```python
from build123d import *

# Parameters (mm, degrees)
TOP_DEPTH             = 5.08
SKETCH2_W             = 5.08
SKETCH2_H             = 44.45
BOLT_ATTACH_DEPTH     = 19.05
BOLTHOLES_LOWER_DEPTH = 5.08
MIRROREDFILLET_R      = 2.54
CENTERFILLET_R        = 6.35
CHAMFER1_SIZE         = 2.54


with BuildPart() as part:
    # Sketch1 → top (new body)
    with BuildSketch(Plane(origin=(0, 0, 0), x_dir=(1, 0, 0), z_dir=(0, 1, 0))):
        Polygon((0, 0), (0, 63.5), (7.62, 63.5), (7.62, 25.4), (17.78, 19.05), (17.78, 0), align=None)
        with BuildLine():
            Line((12.7, 13.97), (12.7, 7.62))
            ThreePointArc((12.7, 7.62), (8.89, 3.81), (5.08, 7.62))
            Line((5.08, 7.62), (5.08, 13.97))
            ThreePointArc((5.08, 13.97), (8.89, 17.78), (12.7, 13.97))
        make_face(mode=Mode.SUBTRACT)
    extrude(amount=TOP_DEPTH)

    # Sketch2 → bolt_attach (add)
    with BuildSketch(Plane.XZ):
        with Locations((2.54, -41.275)):
            Rectangle(SKETCH2_W, SKETCH2_H)
    extrude(amount=BOLT_ATTACH_DEPTH)

    # Sketch3 → boltholes_lower (cut)
    with BuildSketch(Plane(origin=(5.08, 0, 0), x_dir=(0, 0, -1), z_dir=(1, 0, 0))):
        with BuildLine():
            Line((30.48, -3.81), (30.48, -12.7))
            ThreePointArc((30.48, -12.7), (27.305, -15.875), (24.13, -12.7))
            Line((24.13, -12.7), (24.13, -3.81))
            ThreePointArc((24.13, -3.81), (27.305, -0.635), (30.48, -3.81))
        make_face()
        Polygon((63.5, -19.05), (63.5, -12.7), (38.1, -19.05), align=None)
    extrude(amount=-BOLTHOLES_LOWER_DEPTH, mode=Mode.SUBTRACT)

    # mirroredfillet
    mirroredfillet_edges = [part.edges().sort_by_distance(p)[0] for p in [
        (7.62, 2.54, -25.4),
        (17.78, 2.54, -19.05),
        (17.78, 2.54, 0),
        (2.54, -19.05, -19.05),
    ]]
    fillet(mirroredfillet_edges, radius=MIRROREDFILLET_R)

    # Mirror2: part across face


with BuildPart() as part_1:
    add(part.part)
    add(part.part.mirror(Plane(origin=(3.01625, -3.01625, -63.5), x_dir=(1, 0, 0), z_dir=(0, 0, -1))))

    # centerfillet
    centerfillet_edges = [part_1.edges().sort_by_distance(p)[0] for p in [
        (2.54, -12.7, -63.5),
        (2.54, -19.05, -88.9),
        (2.54, -19.05, -38.1),
    ]]
    fillet(centerfillet_edges, radius=CENTERFILLET_R)

    # Chamfer1
    # the kernel refuses this chamfer: 2.54 mm, written as the material it adds along each edge
    with BuildSketch(Plane(origin=(5.08, 0, -19.05), x_dir=(0.9996219169112968, 0.02749587661058638, 0), z_dir=(0, 0, -1))) as chamfer1_piece_1_section:
        Polygon((CHAMFER1_SIZE * 0.999621916911, CHAMFER1_SIZE * 0.0274958766106), (-CHAMFER1_SIZE * 0.0274958766106, CHAMFER1_SIZE * 0.999621916911), (0, 0), align=None)
    chamfer1_piece_1 = extrude(amount=88.9, mode=Mode.PRIVATE)
    chamfer1_piece_1 = chamfer1_piece_1 - Plane(origin=(5.940102797, -3.81, -27.305), x_dir=(0, 0, 1), z_dir=(1, 0, 0)) * Cylinder(3.175, 188, mode=Mode.PRIVATE)
    chamfer1_piece_1 = chamfer1_piece_1 - Plane(origin=(5.940102797, -3.81, -99.695), x_dir=(0, 0, -1), z_dir=(1, 0, 0)) * Cylinder(3.175, 188, mode=Mode.PRIVATE)
    add(chamfer1_piece_1)


solid = part_1.part
```
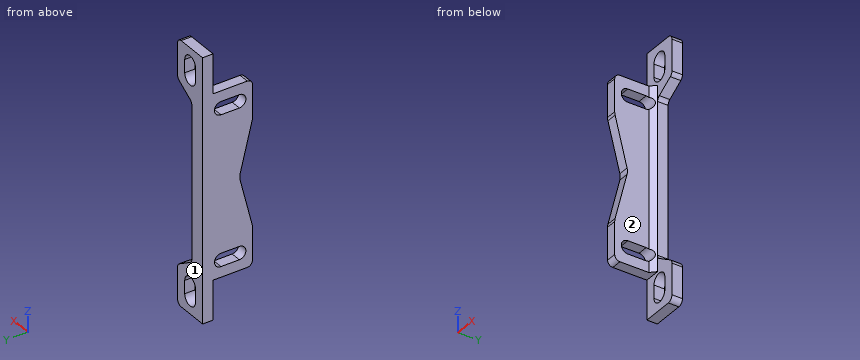
Can you work these out from the model? Positions are in its coordinate system, mm. Face numbers are marked on the shaded views. A direction names the side the tool comes from. Coordinates: 2 decimals unless noted, no trailing zeros. Write each loop counter-clockwise with the first axis right and the second up, starting at its lowest first coordinate (ties: lowest second). Pieces come first, ordered by that corner, then holes. Notation, with made-up numbers: M -11.75,81.25 L 35.25,81.25 A20 ccw 35.25,107.25 Z; hole C 3,25 d10. An arc over 180 degrees is marked long. Write item = value, one per line. Start each with the question number.
Q1. On a 3-axis mill with a long thin cutter (end or side, diameter ignored), from which of +Z, -Z, +X, -X, +Y, -Y can I reach the whole of each face in a straight line? I mean the marked faces 1 and 2. Say none if no direction works.
Q2. If I drill on L1, parallel to Z at x = 1, y = -9; L2, parallel to Z at x = 12.25, y = 1; L3, parallel to Z at x = 9.5, y = 2.5 (3 decimals), over which ranges is the centre line in solid material (lowest first)? Write a range as [from, to].
Q3. I'm going to push flat-ended pins straight in: pin 1 (2.5 mm diameter, centred on x = 1.5, y = -9, fed in from +Z); pin 2 (4 mm diameter, centred on x = 3, y = -8, fed in from -Z); pin 3 (1.5 mm diameter, centred on x = 7, y = -5, fed in from -Z); pin 4 (5.5 mm diameter, centred on x = 13, z = -114, fed in from -Y). Where does each tip first touch, or does it pass through?
Q4. If we section it at B-B, the plane x = 3.75: Write out the boundary of the cut face in (y, z) (3 decimals), then the cut area to 3 significant figures.
Q5. If we section it at D-D, the plane y = 2: Write out the boundary of the cut face in (x, z).
Q6. If we section it at C-C, the plane x = 13.75: Write out the boundary of the cut face in (y, z), then the cut area to 3 significant figures.
Q7. If we section it at A-A, the plane y = -5: Write out the boundary of the cut face in (x, z).
Check sheet entries:
q1.face_1 = +Z, -Z, +X, -X, +Y
q1.face_2 = +Z, -Z, +X, -Y
q2.L1 = [-107.95, -102.87], [-96.52, -30.48], [-24.13, -19.05]
q2.L2 = [-127, -121.18], [-111.23, -104.49], [-22.51, -15.77], [-5.82, 0]
q2.L3 = [-127, -123.141], [-109.269, -102.775], [-24.225, -17.731], [-3.859, 0]
q3.pin_1 = -19.05
q3.pin_2 = -107.95
q3.pin_3 = through
q3.pin_4 = 0
q4.outline = M -19.05,-105.41 A2.54 ccw -16.51,-107.95 L 0,-107.95 L 0,-127 L 5.08,-127 L 5.08,0 L 0,0 L 0,-19.05 L -16.51,-19.05 A2.54 ccw -19.05,-21.59 L -19.05,-37.318 A6.35 ccw -18.86,-38.858 L -13.085,-61.96 A6.35 cw -13.085,-65.04 L -18.86,-88.142 A6.35 ccw -19.05,-89.682 Z; hole M -12.7,-102.87 L -3.81,-102.87 A3.175 ccw -3.81,-96.52 L -12.7,-96.52 A3.175 ccw Z; hole M -12.7,-30.48 L -3.81,-30.48 A3.175 ccw -3.81,-24.13 L -12.7,-24.13 A3.175 ccw Z
q4.area = 2,000 mm²
q5.outline = M 0,-127 L 15.24,-127 A2.54 ccw 17.78,-124.46 L 17.78,-109.36 A2.54 ccw 16.59,-107.2 L 8.81,-102.35 A2.54 cw 7.62,-100.19 L 7.62,-26.81 A2.54 cw 8.81,-24.65 L 16.59,-19.8 A2.54 ccw 17.78,-17.64 L 17.78,-2.54 A2.54 ccw 15.24,0 L 0,0 Z; hole M 5.08,-119.38 A3.81 ccw 12.7,-119.38 L 12.7,-113.03 A3.81 ccw 5.08,-113.03 Z; hole M 5.08,-13.97 A3.81 ccw 12.7,-13.97 L 12.7,-7.62 A3.81 ccw 5.08,-7.62 Z
q6.outline = M 0,-127 L 5.08,-127 L 5.08,-105.43 L 0,-105.43 Z; M 0,-21.57 L 5.08,-21.57 L 5.08,0 L 0,0 Z
q6.area = 219 mm²
q7.outline = M 0,-107.95 L 5.08,-107.95 L 5.08,-102.87 L 0,-102.87 Z; M 0,-96.52 L 5.08,-96.52 L 5.08,-30.48 L 0,-30.48 Z; M 0,-24.13 L 5.08,-24.13 L 5.08,-19.05 L 0,-19.05 Z
